Part model, mm, in its own coordinate system. Face numbers are marked on the shaded views. A direction names the side the tool comes from. Round coordinates to 2 decimals unless told otherwise and drop trailing zeros. Loops run counter-clockwise (first coordinate to the right, second up) from the corner with the lowest first, then second, coordinate; pieces in that order, holes last.
Autodesk Fusion 360 part; units mm, degrees
sketch "Sketch1" plane through (0, 0, 0) normal (0, 0, 1) x (1, 0, 0) in component "Component"
sketch "Sketch1 (2)" plane through (0, 0, 0) normal (0, 0, 1) x (1, 0, 0)
sketch "Sketch2" plane through (0, 0, 0) normal (0, 0, 1) x (1, 0, 0) in component "Component"
  arc A0 (17.6425, 34.6248) -> (62.3575, 34.6248) centre (40, 35) ccw
  arc A1 (23.5355, 34.6248) -> (56.4645, 34.6248) centre (40, 36.7106) ccw
  line L0 (17.6425, 34.6248) -> (23.5355, 34.6248)
  line L1 (56.4645, 34.6248) -> (62.3575, 34.6248)
sketch "Sketch2 (2)" plane through (0, 0, 0) normal (0, 0, 1) x (1, 0, 0)
  line L0 (121.2193, 26.4028) -> (121.2193, 28.2696)
  line L1 (121.2193, 28.2696) -> (121.2193, 58.2696)
  line L2 (161.2193, 58.2696) -> (161.2193, 26.4028)
  line L3 (161.2193, 26.4028) -> (171.2193, 26.4028)
  line L4 (181.2193, 16.4028) -> (101.2193, 16.4028)
  line L5 (121.2193, 26.4028) -> (111.2193, 26.4028)
  line L6 (101.2193, 16.4028) -> (111.2193, 26.4028)
  line L7 (181.2193, 16.4028) -> (171.2193, 26.4028)
  arc A0 (131.2193, 58.2696) -> (151.2193, 58.2696) centre (141.2193, 58.2696) ccw
  arc A1 (121.2193, 58.2696) -> (161.2193, 58.2696) centre (141.2193, 58.2696) ccw
  line L8 (121.2193, 58.2696) -> (131.2193, 58.2696)
  line L9 (151.2193, 58.2696) -> (161.2193, 58.2696)
  dimension "d23" = 20
  dimension "d24" = 20
  dimension "d25" = 40
  dimension "d32" = 80
  dimension "d33" = 10
extrude "Extrude1" add sketch "Sketch2 (2)" along normal blind 40 contours A0 A1 L8 L9
extrude "Extrude2" add sketch "Sketch2 (2)" along normal blind 30 contours L0 L1 L2 L3 L4 L5 L6 L7 A1
component "Component" placed x (1, 0, 0) y (0, 1, 0) z (0, 0, 1) at (0, 0, 0)
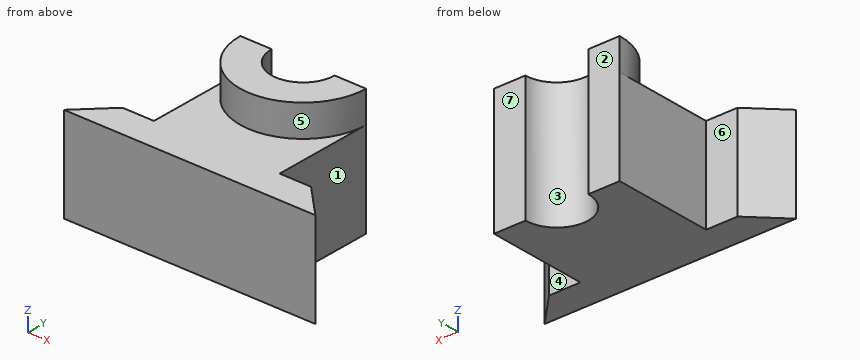
1) Slice it at B-B, the plane z = 16.5. Give the cut face in (x, y).
Values:
outline: (101.22, 16.4) - (181.22, 16.4) - (171.22, 26.4) - (161.22, 26.4) - (161.22, 58.27) - (151.22, 58.27) arc R10 cw to (131.22, 58.27) - (121.22, 58.27) - (121.22, 26.4) - (111.22, 26.4) - close
2) Drop flat-ended pins along their axis: pin 1 Ø1.5 at (y, z) = (46.5, 35.5) entering from +X; pin 2 Ø9 at (y, z) = (34.5, 21.5) entering from +X; pin 3 Ø24 at (y, z) = (45, 9.5) entering from -X. Give the stop position or say it passes through.
Values:
pin 1: stops at x = 157.91
pin 2: stops at x = 161.22
pin 3: stops at x = 121.22
3) Slice it at D-D, the plane x = 137.5. Give the cut face in (y, z).
Values:
outline: (16.4, 0) - (48.99, 0) - (48.99, 40) - (38.62, 40) - (38.62, 30) - (16.4, 30) - close
4) Wall check: line 1 along Z through (x, y) = (132, 24); line 2 along X through (y, z) = (44, 8); line 3 along X through (y, z) = (55.5, 13). Give the ranges that are in metal, low to high.
Values:
line 1: z = 0 to 30
line 2: x = 121.22 to 161.22
line 3: x = 121.22 to 131.61, 150.83 to 161.22
5) Slice it at A-A, the plane y = 49.5. Give the cut face in (x, z).
Values:
outline: (121.22, 0) - (136.41, 0) - (136.41, 40) - (123.24, 40) - (123.24, 30) - (121.22, 30) - close; (146.02, 0) - (161.22, 0) - (161.22, 30) - (159.19, 30) - (159.19, 40) - (146.02, 40) - close
6) Tool access for the marked faces 4, 5, 6 and 7: list every direction of +Z, -Z, +X, -X, +Y, -Y with a clear straight run to the whole face (end or side of a thin tool).
Values:
face 4: +Z, -Z, +X, +Y
face 5: +Z, -Y
face 6: +Z, -Z, -X, +Y
face 7: +Z, -Z, +X, -X, +Y
7) Slice it at C-C, the plane y = 40. Give the cut face in (x, z), then the cut area to 3 significant figures.
Values:
outline: (121.22, 0) - (161.22, 0) - (161.22, 30) - (149.36, 30) - (149.36, 40) - (133.08, 40) - (133.08, 30) - (121.22, 30) - close
area: 1,360 mm2
8) Mould opens along X. For the marked faces 1, 2 and 3 say: released by +X, released by -X, zero draft, split by the parting line, or undercut.
Values:
face 1: released by +X
face 2: zero draft
face 3: undercut
